For this review, take the finished solid that the model builds, in its own axes (mm). A direction names the side the tool comes from. Round coordinates to 2 decimals unless told otherwise and drop trailing zeros. Order: outer loops, then holes, each group sorted by start corner. A loop starts at its lowest first (then second) coordinate and runs counter-clockwise, first axis right, second up. Notation, with made-up numbers: M 87,-25.5 L 133,-25.5 A28 ccw 133,-3.5 Z; hole C -9.5,77 d6. An arc over 180 degrees is marked long. Answer as a JSON object with one key per item and string values.
from build123d import *

# Parameters (mm, degrees)
BOSS_EXTRUDE1_DEPTH = 2.5
SKETCH2_R           = 6.35
BOSS_EXTRUDE2_DEPTH = 18.5
SKETCH3_R           = 5.5
CUT_EXTRUDE3_DEPTH  = 18.5
SKETCH4_R           = 5
CUT_EXTRUDE4_DEPTH  = 27.752756867
FILLET1_R           = 0.75


with BuildPart() as part:
    # Sketch1 → Boss-Extrude1 (new body)
    with BuildSketch(Plane.XY):
        Polygon((8.5, 0), (4.25, 7.361215932), (-4.25, 7.361215932), (-8.5, 0), (-4.25, -7.361215932), (4.25, -7.361215932), align=None)
    extrude(amount=BOSS_EXTRUDE1_DEPTH)

    # Sketch2 → Boss-Extrude2 (add)
    with BuildSketch(Plane.XY.offset(2.5)):
        Circle(SKETCH2_R)
    extrude(amount=BOSS_EXTRUDE2_DEPTH)

    # Sketch3 → Cut-Extrude3 (cut)
    with BuildSketch(Plane.XY.offset(21)):
        Circle(SKETCH3_R)
    extrude(amount=-CUT_EXTRUDE3_DEPTH, mode=Mode.SUBTRACT)

    # Sketch4 → Cut-Extrude4 (cut, through all)
    with BuildSketch(Plane.ZY.offset(6.35)):
        with Locations(Location((11, 0, 0), (0, 0, 270))):
            Circle(SKETCH4_R)
    extrude(amount=-CUT_EXTRUDE4_DEPTH, mode=Mode.SUBTRACT)

    # Fillet1
    fillet1_edges = [part.edges().sort_by_distance(p)[0] for p in [
        (4.25, -7.361215932, 1.25),
        (-4.25, -7.361215932, 1.25),
        (-8.5, 0, 1.25),
        (-4.25, 7.361215932, 1.25),
        (4.25, 7.361215932, 1.25),
        (8.5, 0, 1.25),
    ]]
    fillet(fillet1_edges, radius=FILLET1_R)


solid = part.part
1) Add section D-D on x = 5.25. State the section outline as (y, z) points, and give its area (3 significant figures).
Geometry check:
{"outline": "M -5.63,0 L 5.63,0 L 5.63,2.5 L 3.57,2.5 L 3.57,7.5 A5 cw 1.64,6.28 L 1.64,2.5 L -1.64,2.5 L -1.64,6.28 A5 cw -3.57,7.5 L -3.57,2.5 L -5.63,2.5 Z; M -3.57,14.5 A5 cw -1.64,15.72 L -1.64,21 L -3.57,21 Z; M 1.64,15.72 A5 cw 3.57,14.5 L 3.57,21 L 1.64,21 Z", "area": "67.1 mm²"}
2) Insertion check: P1, Ø4, axis at x = -5.5, z = 13, coming from the -Y side; P2, Ø4, axis at y = -2.5, z = 13, coming from the -X side; P3, Ø4, axis at y = 1.5, z = 18.5, coming from the -X side. Each pin has a flat end and moves straight along its axis. Give the tip position at first contact, or say it passes through.
Geometry check:
{"P1": "stops at y = -5.3", "P2": "stops at x = -5.52", "P3": "stops at x = -6.35"}
3) Add section C-C on z = 10.25. State the section outline as (x, y) points, and give its area (3 significant figures).
Geometry check:
{"outline": "M -3.99,-4.94 A6.35 ccw 3.99,-4.94 L 2.41,-4.94 A5.5 cw -2.41,-4.94 Z; M -3.99,4.94 L -2.41,4.94 A5.5 cw 2.41,4.94 L 3.99,4.94 A6.35 ccw Z", "area": "11.7 mm²"}
4) Mouldability with a two-part tool opening along Y and no side actions: class faces 3 (the flat face through (-6.402, -3.634, 1.232)), 4 (the flat face through (6.402, 3.634, 1.232)), 5 (the cylindrical face through (-4, -4, 14)), 6 (the cylindrical face through (-1.19, -5.37, 11.88)) as +Y half, -Y half, draft (parallel to the pull), parting line (faces both ways), or undercut.
Geometry check:
{"face 3": "-Y half", "face 4": "+Y half", "face 5": "undercut", "face 6": "undercut"}
5) Machinability: for faces 1 (the flat face through (-5, 3, 21)), 2 (the flat face through (0, 0, 2.5)), which of the approach directions +Z, -Z, +X, -X, +Y, -Y give a long, thin tool a straight path to every point of the face, cutting with its end or side? Answer none if there is none.
Geometry check:
{"face 1": "+Z, +X, -X, +Y, -Y", "face 2": "+Z"}
6) Add section A-A on y = 0. State the section outline as (x, z) points, and give its area (3 significant figures).
Geometry check:
{"outline": "M -8.38,0 L 8.38,0 L 8.38,2.5 L 6.35,2.5 L 6.35,6 L 5.5,6 L 5.5,2.5 L -5.5,2.5 L -5.5,6 L -6.35,6 L -6.35,2.5 L -8.38,2.5 Z; M -6.35,16 L -5.5,16 L -5.5,21 L -6.35,21 Z; M 5.5,16 L 6.35,16 L 6.35,21 L 5.5,21 Z", "area": "56.4 mm²"}
7) For L1, parallel to Y at x = -0.25, z = 12; L2, parallel to Z at x = 0.5, y = -5; L3, parallel to X at y = 0.75, z = 5.75, list the stretches that pass through material, from the lowest coordinate up.
Geometry check:
{"L1": "y = -6.35 to -5.49, 5.49 to 6.35", "L2": "z = 0 to 2.5", "L3": "x = -6.31 to -5.45, 5.45 to 6.31"}
8) Add section B-B on x = 0. State the section outline as (y, z) points, and give its area (3 significant figures).
Geometry check:
{"outline": "M -7.36,0 L 7.36,0 L 7.36,2.5 L 6.35,2.5 L 6.35,21 L 5.5,21 L 5.5,2.5 L -5.5,2.5 L -5.5,21 L -6.35,21 L -6.35,2.5 L -7.36,2.5 Z", "area": "68.3 mm²"}
